Verification items for the finished model (mm, model axes). A direction names the side the tool comes from. Coordinates: 2 decimals unless noted, no trailing zeros. Write each loop counter-clockwise with the first axis right and the second up, starting at its lowest first coordinate (ties: lowest second). Pieces come first, ordered by that corner, then holes. Notation, with made-up numbers: M -7.75,31 L 4.25,31 A10 cw 4.25,35 Z; hole C -19,68.25 d10. An arc over 180 degrees is marked long. Answer in a Markdown table with one row per item.
from build123d import *

# Parameters (mm, degrees)
BOSS_EXTRUDE1_DEPTH     = 3
CUT_EXTRUDE2_DEPTH      = 180.232477503
CUT_EXTRUDE2_DEPTH_BACK = 3


with BuildPart() as part:
    # Sketch1 → Boss-Extrude1 (new body)
    with BuildSketch(Plane(origin=(0, 0, 0), x_dir=(0, 0, -1), z_dir=(1, 0, 0))):
        Polygon((-169.090909091, 50), (-139.090909091, 50), (-139.090909091, 47), (100.909090909, 47), (100.909090909, 50), (130.909090909, 50), (130.909090909, 30), (133.909090909, 30), (133.909090909, 0), (130.909090909, 0), (130.909090909, -10), (-169.090909091, -10), (-169.090909091, 0), (-172.090909091, 0), (-172.090909091, 30), (-169.090909091, 30), align=None)
    extrude(amount=BOSS_EXTRUDE1_DEPTH)

    # Sketch2 → Cut-Extrude2 (cut, two sides: drawn at the far end of the back side and taken through both)
    with BuildSketch(Plane.ZY.offset(-CUT_EXTRUDE2_DEPTH_BACK)):
        with BuildLine():
            Line((-100.909090909, -579.031305027), (-100.909090909, -10))
            Line((-100.909090909, -10), (-100.909090909, 15.818953756))
            ThreePointArc((-100.909090909, 15.818953756), (-99.444624815, 19.354487662), (-95.909090909, 20.818953756))
            Line((-95.909090909, 20.818953756), (134.090909091, 20.818953756))
            ThreePointArc((134.090909091, 20.818953756), (137.626442997, 19.354487662), (139.090909091, 15.818953756))
            Line((139.090909091, 15.818953756), (139.090909091, -10))
            Line((139.090909091, -10), (139.090909091, -579.031305027))
            Line((139.090909091, -579.031305027), (139.090909091, -1717.09391508))
            Line((139.090909091, -1717.09391508), (-100.909090909, -1717.09391508))
            Line((-100.909090909, -1717.09391508), (-100.909090909, -579.031305027))
        make_face()
    extrude(amount=CUT_EXTRUDE2_DEPTH + CUT_EXTRUDE2_DEPTH_BACK, mode=Mode.SUBTRACT)


solid = part.part
1) Tool access check on faces 3 (the face through (1.52, 19.39, 137.59)), 4 (the face through (0, 27, 17)). Record the directions out of +Z, -Z, +X, -X, +Y, -Y that give a thin tool (end or side, any length) a straight path to the whole face; none if there is none.
Response values:
| item | result |
|---|---|
| face 3 | +X, -X, -Y |
| face 4 | +Z, -Z, -X, +Y, -Y |
2) Thickness scan on L1, parallel to Z at x = 0.95, y = -2.5; L2, parallel to Z at x = 0.85, y = 13.5; L3, parallel to Y at x = 2.6, z = 114. Record the ranges inside material, lowest first. Write a range as [from, to].
Response values:
| item | result |
|---|---|
| L1 | z = [-130.91, -100.91], [139.09, 169.09] |
| L2 | z = [-133.91, -100.91], [139.09, 172.09] |
| L3 | y = [20.82, 47] |
3) Sectioned sample at C-C (y = -3). Record the cut outline in (x, z), then the cut area to 3 significant figures.
Response values:
| item | result |
|---|---|
| outline | M 0,-130.91 L 3,-130.91 L 3,-100.91 L 0,-100.91 Z; M 0,139.09 L 3,139.09 L 3,169.09 L 0,169.09 Z |
| area | 180 mm² |
4) Sectioned sample at A-A (y = 10). Record the cut outline in (x, z), then the cut area to 3 significant figures.
Response values:
| item | result |
|---|---|
| outline | M 0,-133.91 L 3,-133.91 L 3,-100.91 L 0,-100.91 Z; M 0,139.09 L 3,139.09 L 3,172.09 L 0,172.09 Z |
| area | 198 mm² |
5) Depth check by flat-ended pin: pin 1 (1.5 mm diameter, centred on x = 2, y = -5, fed in from -Z); pin 2 (1.5 mm diameter, centred on x = 2, y = 49, fed in from +Z); pin 3 (1.5 mm diameter, centred on x = 2, z = -132.5, fed in from +Y); pin 4 (8 mm diameter, centred on y = 16, z = 70.5, fed in from +X). Enter the tip coordinate at first touch or a pass-through.
Response values:
| item | result |
|---|---|
| pin 1 | stops at z = -130.91 |
| pin 2 | stops at z = 169.09 |
| pin 3 | stops at y = 30 |
| pin 4 | passes through |
6) Release check for a two-part mould opening along Z. For faces 1 (the face through (3, 27, 17)), 2 (the face through (1.5, 19.3, -99.5)) record: +Z half, -Z half, draft (parallel to the pull), parting line (faces both ways), or undercut.
Response values:
| item | result |
|---|---|
| face 1 | draft |
| face 2 | undercut |
7) Sectioned sample at B-B (x = 1.25). Record the cut outline in (y, z), then the cut area to 3 significant figures.
Response values:
| item | result |
|---|---|
| outline | M -10,-130.91 L 0,-130.91 L 0,-133.91 L 30,-133.91 L 30,-130.91 L 50,-130.91 L 50,-100.91 L 47,-100.91 L 47,139.09 L 50,139.09 L 50,169.09 L 30,169.09 L 30,172.09 L 0,172.09 L 0,169.09 L -10,169.09 L -10,139.09 L 15.82,139.09 A5 cw 20.82,134.09 L 20.82,-95.91 A5 cw 15.82,-100.91 L -10,-100.91 Z |
| area | 10,100 mm² |
8) Sectioned sample at D-D (z = 2). Record the cut outline in (x, y).
Response values:
| item | result |
|---|---|
| outline | M 0,20.82 L 3,20.82 L 3,47 L 0,47 Z |
